```python
from build123d import *

# Parameters (mm, degrees)
SKETCH1_R        = 1.5
SKETCH1_R_2      = 1.6
SKETCH1_R_3      = 2
SKETCH1_R_4      = 1.35
SKETCH1_W        = 22
SKETCH1_H        = 3.516266508
EXTRUSION1_DEPTH = 1.6
FILLET1_R        = 1
FILLET2_R        = 4
FILLET3_R        = 3
FILLET4_R        = 3
FILLET5_R        = 2
FILLET6_R        = 2
FILLET7_R        = 3
FILLET8_R        = 3
FILLET9_R        = 2
FILLET10_R       = 2
FILLET11_R       = 3


with BuildPart() as part:
    # Sketch1 → Extrusion1 (new body)
    with BuildSketch(Plane(origin=(0, 0, 0), x_dir=(-1, 0, 0), z_dir=(0, 1, 0))):
        Polygon((59.775158519, 259.059874387), (56.775158519, 264.05987395), (36.775158519, 264.05987395), (36.775158519, 252.05987395), (18.755330752, 234.731117294), (21.527931817, 231.847944851), (10.275158581, 204.559863083), (7.275158519, 204.559863083), (7.275158519, 183.059873956), (7.275158519, 161.559884829), (10.275158581, 161.559884829), (21.527931817, 134.27180306), (18.755330752, 131.388630617), (36.775158519, 114.059873961), (36.775158519, 102.059873961), (56.775158519, 102.059873961), (59.775158519, 107.059873524), (76.297476624, 107.059873524), (95.297476624, 107.059873524), (98.297476624, 102.059873961), (118.297476624, 102.059873961), (118.297476624, 114.059873961), (136.317304391, 131.388630617), (133.544703326, 134.27180306), (144.797476562, 161.559884829), (150.275158519, 161.559884829), (150.275158519, 183.059873956), (150.275158519, 204.559863083), (147.275158457, 204.559863083), (136.022385221, 231.847944851), (137.604565953, 233.493222978), (118.297476624, 252.05987395), (118.297476624, 264.05987395), (98.297476624, 264.05987395), (95.297476624, 259.059874387), (76.297476624, 259.059874387), align=None)
        with Locations(Location((55.775158457, 111.059872631, 0), (0, 0, 90))):
            Circle(SKETCH1_R, mode=Mode.SUBTRACT)
        with Locations(Location((39.275158457, 118.059884829, 0), (0, 0, 90))):
            Circle(SKETCH1_R, mode=Mode.SUBTRACT)
        with Locations(Location((17.275158457, 174.809872631, 0), (0, 0, 90))):
            Circle(SKETCH1_R_2, mode=Mode.SUBTRACT)
        with Locations(Location((76.297476624, 183.059873956, 0), (0, 0, 90))):
            Circle(SKETCH1_R_3, mode=Mode.SUBTRACT)
        with Locations(Location((41.775158457, 255.059863083, 0), (0, 0, 90))):
            Circle(SKETCH1_R, mode=Mode.SUBTRACT)
        with Locations(Location((39.275158457, 248.059863083, 0), (0, 0, 90))):
            Circle(SKETCH1_R, mode=Mode.SUBTRACT)
        with Locations(Location((10.775158457, 194.05987528, 0), (0, 0, 90))):
            Circle(SKETCH1_R_4, mode=Mode.SUBTRACT)
        with Locations(Location((88.775158581, 111.059872631, 0), (0, 0, 90))):
            Circle(SKETCH1_R, mode=Mode.SUBTRACT)
        with Locations(Location((115.775158581, 111.059884829, 0), (0, 0, 90))):
            Circle(SKETCH1_R, mode=Mode.SUBTRACT)
        with Locations(Location((118.275158581, 118.059884829, 0), (0, 0, 90))):
            Circle(SKETCH1_R, mode=Mode.SUBTRACT)
        with Locations(Location((140.275158581, 174.809872631, 0), (0, 0, 90))):
            Circle(SKETCH1_R_2, mode=Mode.SUBTRACT)
        with Locations(Location((115.775158581, 255.059863083, 0), (0, 0, 90))):
            Circle(SKETCH1_R, mode=Mode.SUBTRACT)
        with Locations(Location((88.775158581, 254.309863083, 0), (0, 0, 90))):
            Circle(SKETCH1_R, mode=Mode.SUBTRACT)
        with Locations(Location((140.275158581, 191.30987528, 0), (0, 0, 90))):
            Circle(SKETCH1_R_2, mode=Mode.SUBTRACT)
        with Locations(Location((146.775158581, 194.05987528, 0), (0, 0, 90))):
            Circle(SKETCH1_R_4, mode=Mode.SUBTRACT)
        with Locations(Location((101.775158581, 254.309863083, 0), (0, 0, 90))):
            Circle(SKETCH1_R, mode=Mode.SUBTRACT)
        with Locations(Location((118.275158581, 248.059863083, 0), (0, 0, 90))):
            Circle(SKETCH1_R, mode=Mode.SUBTRACT)
        with Locations(Location((146.775158581, 172.059872631, 0), (0, 0, 90))):
            Circle(SKETCH1_R_4, mode=Mode.SUBTRACT)
        with Locations(Location((101.775158581, 111.059872631, 0), (0, 0, 90))):
            Circle(SKETCH1_R, mode=Mode.SUBTRACT)
        with Locations(Location((17.275158457, 191.30987528, 0), (0, 0, 90))):
            Circle(SKETCH1_R_2, mode=Mode.SUBTRACT)
        with Locations(Location((55.775158457, 254.309863083, 0), (0, 0, 90))):
            Circle(SKETCH1_R, mode=Mode.SUBTRACT)
        with Locations(Location((68.775158457, 254.309863083, 0), (0, 0, 90))):
            Circle(SKETCH1_R, mode=Mode.SUBTRACT)
        with Locations(Location((10.775158457, 172.059872631, 0), (0, 0, 90))):
            Circle(SKETCH1_R_4, mode=Mode.SUBTRACT)
        with Locations(Location((68.775158457, 111.059872631, 0), (0, 0, 90))):
            Circle(SKETCH1_R, mode=Mode.SUBTRACT)
        with Locations(Location((41.775158457, 111.059884829, 0), (0, 0, 90))):
            Circle(SKETCH1_R, mode=Mode.SUBTRACT)
        with Locations(Location((32.775158457, 124.309884829, 0), (0, 0, 90))):
            Circle(SKETCH1_R, mode=Mode.SUBTRACT)
        with Locations(Location((124.775158581, 241.809863083, 0), (0, 0, 90))):
            Circle(SKETCH1_R, mode=Mode.SUBTRACT)
        with Locations(Location((32.775158457, 241.809863083, 0), (0, 0, 90))):
            Circle(SKETCH1_R, mode=Mode.SUBTRACT)
        with Locations(Location((124.775158581, 124.309884829, 0), (0, 0, 90))):
            Circle(SKETCH1_R, mode=Mode.SUBTRACT)
        with Locations((61.297476624, 183.059873956)):
            Rectangle(SKETCH1_W, SKETCH1_H, mode=Mode.SUBTRACT)
        with Locations((91.297476624, 183.059873956)):
            Rectangle(SKETCH1_W, SKETCH1_H, mode=Mode.SUBTRACT)
    extrude(amount=EXTRUSION1_DEPTH)

    # Fillet1
    fillet1_edges = [part.edges().sort_by_distance(p)[0] for p in [
        (-95.297476624, 0.8, 259.059874387),
        (-95.297476624, 0.8, 107.059873524),
        (-59.775158519, 0.8, 107.059873524),
        (-59.775158519, 0.8, 259.059874387),
    ]]
    fillet(fillet1_edges, radius=FILLET1_R)

    # Fillet2
    fillet2_edges = [part.edges().sort_by_distance(p)[0] for p in [
        (-118.297476624, 0.8, 264.05987395),
        (-118.297476624, 0.8, 102.059873961),
        (-36.775158519, 0.8, 102.059873961),
        (-36.775158519, 0.8, 264.05987395),
    ]]
    fillet(fillet2_edges, radius=FILLET2_R)

    # Fillet3
    fillet3_edges = [part.edges().sort_by_distance(p)[0] for p in [
        (-118.297476624, 0.8, 252.05987395),
        (-118.297476624, 0.8, 114.059873961),
        (-36.775158519, 0.8, 114.059873961),
        (-36.775158519, 0.8, 252.05987395),
    ]]
    fillet(fillet3_edges, radius=FILLET3_R)

    # Fillet4
    # the kernel refuses this fillet: 3 mm, written as the material it takes off along each edge
    with BuildSketch(Plane(origin=(-137.604565953, -7.282396937, 233.493222978), x_dir=(0.7207931106757886, 0, 0.6931502662499095), z_dir=(0, 1, 0))) as fillet4_piece_1:
        with BuildLine():
            CenterArc((2.912958775, 3), FILLET4_R, 193.835510016, 76.164489984)
            Line((0, 2.282594135), (-0.058259176, 2.268246017))
            ThreePointArc((-0.058259176, 2.268246017), (-0.06, 1.141297067), (-0.06, 0))
            Line((-0.06, 0), (0, -0.06))
            Line((0, -0.06), (2.912958775, -0.06))
            Line((2.912958775, -0.06), (2.912958775, 0))
        make_face()
    extrude(amount=16.164793875, mode=Mode.SUBTRACT)

    # Fillet5
    fillet5_edges = [part.edges().sort_by_distance(p)[0] for p in [
        (-136.022385221, 0.8, 231.847944851),
    ]]
    fillet(fillet5_edges, radius=FILLET5_R)

    # Fillet6
    fillet6_edges = [part.edges().sort_by_distance(p)[0] for p in [
        (-21.527931817, 0.8, 231.847944851),
    ]]
    fillet(fillet6_edges, radius=FILLET6_R)

    # Fillet7
    fillet7_edges = [part.edges().sort_by_distance(p)[0] for p in [
        (-18.755330752, 0.8, 234.731117294),
    ]]
    fillet(fillet7_edges, radius=FILLET7_R)

    # Fillet8
    fillet8_edges = [part.edges().sort_by_distance(p)[0] for p in [
        (-136.317304391, 0.8, 131.388630617),
        (-18.755330752, 0.8, 131.388630617),
    ]]
    fillet(fillet8_edges, radius=FILLET8_R)

    # Fillet9
    fillet9_edges = [part.edges().sort_by_distance(p)[0] for p in [
        (-21.527931817, 0.8, 134.27180306),
        (-133.544703326, 0.8, 134.27180306),
    ]]
    fillet(fillet9_edges, radius=FILLET9_R)

    # Fillet10
    fillet10_edges = [part.edges().sort_by_distance(p)[0] for p in [
        (-147.275158457, 0.8, 204.559863083),
        (-144.797476562, 0.8, 161.559884829),
        (-10.275158581, 0.8, 161.559884829),
        (-10.275158581, 0.8, 204.559863083),
    ]]
    fillet(fillet10_edges, radius=FILLET10_R)

    # Fillet11
    fillet11_edges = [part.edges().sort_by_distance(p)[0] for p in [
        (-150.275158519, 0.8, 161.559884829),
        (-150.275158519, 0.8, 204.559863083),
        (-7.275158519, 0.8, 204.559863083),
        (-7.275158519, 0.8, 161.559884829),
    ]]
    fillet(fillet11_edges, radius=FILLET11_R)


solid = part.part
```
Read the model definition and answer for the solid it produces. Units are mm, in the model's axes. Coordinates: 2 decimals unless noted, no trailing zeros. Write each loop counter-clockwise with the first axis right and the second up, starting at its lowest first coordinate (ties: lowest second). Pieces come first, ordered by that corner, then holes. Notation, with made-up numbers: (-31, 19) - (8, 19) arc R32 cw to (8, 53) - close; hole circle Ø2 at (28, 21). An arc over 180 degrees is marked (long way). Answer as a JSON object with one key per item and string values. Group by question number.
1. A cutting plane is placed at B-B (x = -29.5). Determine the outline of the cut face in (y, z).
2. A cutting plane is placed at C-C (z = 150.5). Determine the outline of the cut face in (x, y), plus the area to 3 significant figures.
3. Consider L1, parallel to Z at x = -92.5, y = 1.2; L2, parallel to X at y = 0.4, z = 182.5; L3, parallel to X at y = 1.3, z = 172. Determine where each line is inside the solid, lowest interval first. Write a range as [from, to].
4. The mould has two halves that part along Z. Classify faces 1 (the cylindrical face through (-77.51, 0.79, 181.47)), 2 (the flat face through (-78, 1.6, 166)), 3 (the flat face through (-127.48, 0.79, 243.23)): +Z half, -Z half, draft (parallel to the pull), parting line (faces both ways), or undercut.
5. A cutting plane is placed at A-A (y = 1.2). Give the number of separate pieces and of enclosed holes in the cut face, plus the area to 3 significant figures.
Worked out:
{
 "1": {"outline": "(0, 121.06) - (1.6, 121.06) - (1.6, 245.06) - (0, 245.06) - close"},
 "2": {"outline": "(-140.24, 0) - (-14.84, 0) - (-14.84, 1.6) - (-140.24, 1.6) - close", "area": "201 mm²"},
 "3": {"L1": "z = [107.06, 181.3], [184.82, 259.06]", "L2": "x = [-150.28, -102.3], [-80.3, -78.22], [-74.38, -72.3], [-50.3, -7.28]", "L3": "x = [-150.28, -148.12], [-145.43, -12.12], [-9.43, -7.28]"},
 "4": {"face 1": "undercut", "face 2": "draft", "face 3": "+Z half"},
 "5": {"separate pieces": "1", "enclosed holes": "31", "area": "18,200 mm²"}
}
